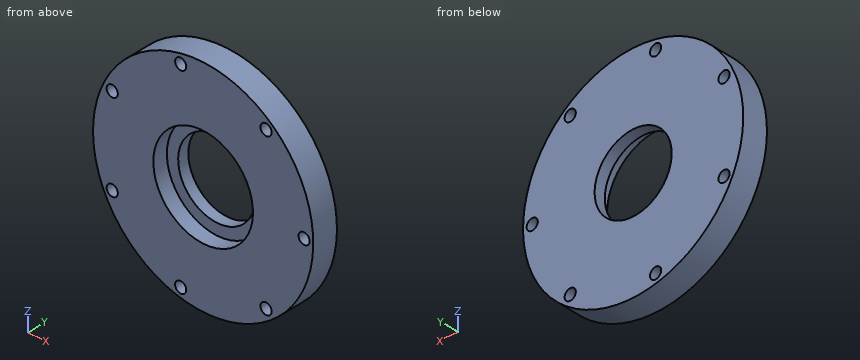
from build123d import *

# Parameters (mm, degrees)
CROQUIS1_R              = 30
CROQUIS1_R_2            = 10.5
SALIENTE_EXTRUIR1_DEPTH = 7
CROQUIS2_R              = 13.575
CORTAR_EXTRUIR1_DEPTH   = 4
CROQUIS3_R              = 1.52
CORTAR_EXTRUIR2_DEPTH   = 44


with BuildPart() as part:
    # Croquis1 → Saliente-Extruir1 (new body)
    with BuildSketch(Plane(origin=(0, 0, 0), x_dir=(1, 0, 0), z_dir=(0, 1, 0))):
        with Locations(Location((0, 0, 0), (0, 0, 270))):
            Circle(CROQUIS1_R)
        with Locations(Location((0, 0, 0), (0, 0, 270))):
            Circle(CROQUIS1_R_2, mode=Mode.SUBTRACT)
    extrude(amount=SALIENTE_EXTRUIR1_DEPTH)

    # Croquis2 → Cortar-Extruir1 (cut)
    with BuildSketch(Plane.XZ):
        with Locations(Location((0, 0, 0), (0, 0, 270))):
            Circle(CROQUIS2_R)
    extrude(amount=-CORTAR_EXTRUIR1_DEPTH, mode=Mode.SUBTRACT)

    # Croquis3 → Cortar-Extruir2 (cut, through all)
    with BuildSketch(Plane(origin=(0, 7, 0), x_dir=(1, 0, 0), z_dir=(0, 1, 0))):
        with Locations(Location((27.5, 0, 0), (0, 0, 270))):
            Circle(CROQUIS3_R)
        with Locations(Location((17.145969551, -21.500365768, 0), (0, 0, 270))):
            Circle(CROQUIS3_R)
        with Locations(Location((-6.119325684, -26.810517585, 0), (0, 0, 270))):
            Circle(CROQUIS3_R)
        with Locations(Location((-24.776643867, -11.931802826, 0), (0, 0, 270))):
            Circle(CROQUIS3_R)
        with Locations(Location((-24.776643867, 11.931802826, 0), (0, 0, 270))):
            Circle(CROQUIS3_R)
        with Locations(Location((-6.119325684, 26.810517585, 0), (0, 0, 270))):
            Circle(CROQUIS3_R)
        with Locations(Location((17.145969551, 21.500365768, 0), (0, 0, 270))):
            Circle(CROQUIS3_R)
    extrude(amount=-CORTAR_EXTRUIR2_DEPTH, mode=Mode.SUBTRACT)


solid = part.part
Here's how the part is built. I have some questions about the finished solid (model axes, mm). Round coordinates to 2 decimals unless told otherwise and drop trailing zeros. Write each loop counter-clockwise with the first axis right and the second up, starting at its lowest first coordinate (ties: lowest second). Pieces come first, ordered by that corner, then holes. Notation, with made-up numbers: (3.25, 85.25) -> (25.25, 85.25) arc R10 cw to (25.25, 97.25) -> close; hole circle Ø10 at (75, 12.25). An arc over 180 degrees is marked (long way). One line per item, written item: value.
1) Suppose I cut it at B-B on z = 0. List the corners of the cut face in (x, y) for me (3 decimals), plus the area to 3 significant figures.
Filled sheet:
outline: (-30, 0) -> (-13.575, 0) -> (-13.575, 4) -> (-10.5, 4) -> (-10.5, 7) -> (-30, 7) -> close; (10.5, 4) -> (13.575, 4) -> (13.575, 0) -> (25.98, 0) -> (25.98, 7) -> (10.5, 7) -> close; (29.02, 0) -> (30, 0) -> (30, 7) -> (29.02, 7) -> close
area: 227 mm2
2) Suppose I cut it at D-D on x = 24. List the corners of the cut face in (y, z) for me, plus the area to 3 significant figures.
Filled sheet:
outline: (0, -18) -> (7, -18) -> (7, 18) -> (0, 18) -> close
area: 252 mm2
3) If I drill on line 1 (X direction, y = 2, z = 0) (3 decimals); line 2 (X direction, y = 5.7, z = 0); line 3 (Z direction, x = 18.5, y = 3.75), over which ranges is the centre line in solid material (lowest first)? Write a range as [from, to].
Filled sheet:
line 1: x = [-30, -13.575], [13.575, 25.98], [29.02, 30]
line 2: x = [-30, -10.5], [10.5, 25.98], [29.02, 30]
line 3: z = [-23.62, -22.19], [-20.81, 20.81], [22.19, 23.62]
4) Suppose I cut it at A-A on x = 0. List the corners of the cut face in (y, z) for me (3 decimals).
Filled sheet:
outline: (0, -30) -> (7, -30) -> (7, -10.5) -> (4, -10.5) -> (4, -13.575) -> (0, -13.575) -> close; (0, 13.575) -> (4, 13.575) -> (4, 10.5) -> (7, 10.5) -> (7, 30) -> (0, 30) -> close
5) I'm going to push flat-ended pins straight in: pin 1 Ø1.8 at (x, z) = (-24.78, -11.93) entering from -Y; pin 2 Ø13.5 at (x, z) = (5.5, 0) entering from -Y; pin 3 Ø1.5 at (x, y) = (16, 4) entering from -Z; pin 4 Ø4 at (x, z) = (-6.12, 26.81) entering from -Y. Where does each tip first touch, or does it pass through?
Filled sheet:
pin 1: passes through
pin 2: stops at y = 4
pin 3: stops at z = -25.83
pin 4: stops at y = 0
6) Suppose I cut it at C-C on y = 3. Give the number of separate pieces and of enclosed holes in the cut face, plus the area to 3 significant figures.
Filled sheet:
separate pieces: 1
enclosed holes: 8
area: 2,200 mm2
